Design review of the part shown in the three views and the two pictorial views. Dimensions are in mm from the part's minimum x, y and z. Round coordinates to 2 decimals unless told otherwise and drop trailing zeros. Loops run counter-clockwise (first coordinate to the right, second up) from the corner with the lowest first, then second, coordinate; pieces in that order, holes last.
1. Consider section B-B on x = 12.7. State the section outline as (y, z) points.
2. Clearance check with a flat-ended pin moving along its axis: pin 1 Ø4 at (x, y) = (63.5, 12.7) entering from -Z. State where the tip first meets the part, or that it passes through.
3. Consider section A-A on y = 38.1. State the section outline as (x, z) points.
4. To check wall thickness, follow line 1 along Y through (x, z) = (38.1, 2.5); line 2 along Y through (x, z) = (10, 0.75) (1 decimal); line 3 along X through (y, z) = (13.5, 1.75). State the ranges of each line that lie inside material, in increasing order.
5. Consider section D-D on z = 1. State how many separate pieces and enclosed holes the cut face has, then the cut area to 3 significant figures.
6. Consider section C-C on y = 63.5. State the section outline as (x, z) points.
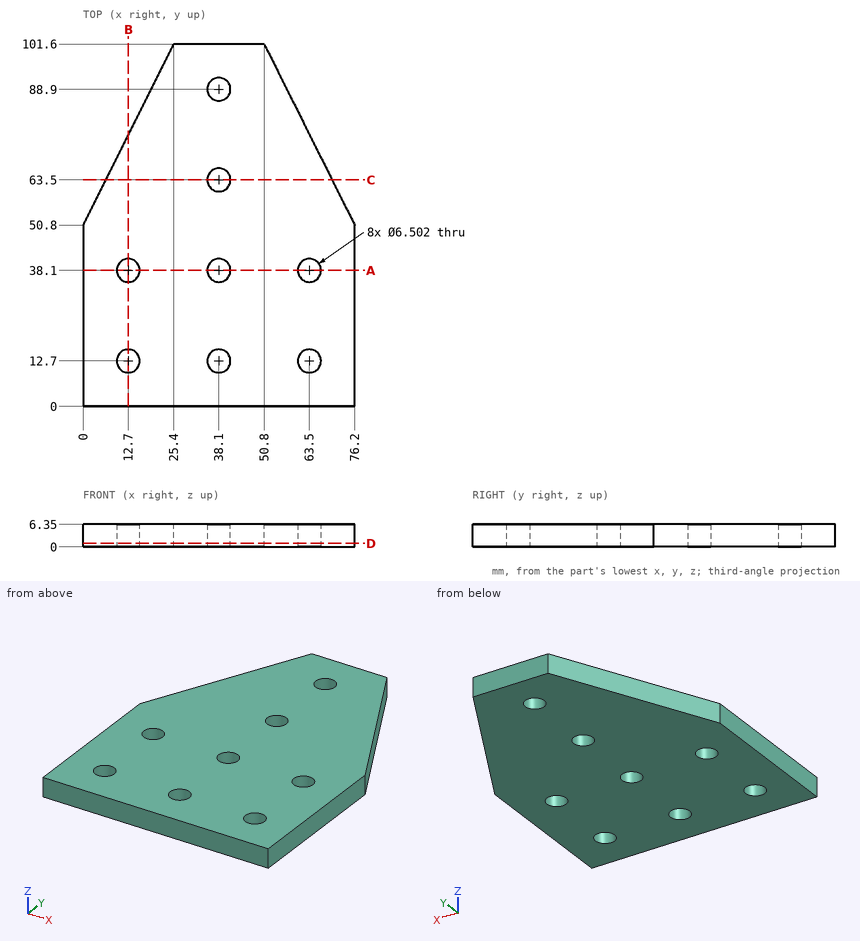
Resolved:
1. outline: (0, 0) - (9.45, 0) - (9.45, 6.35) - (0, 6.35) - close; (15.95, 0) - (34.85, 0) - (34.85, 6.35) - (15.95, 6.35) - close; (41.35, 0) - (76.2, 0) - (76.2, 6.35) - (41.35, 6.35) - close
2. pin 1: passes through
3. outline: (0, 0) - (9.45, 0) - (9.45, 6.35) - (0, 6.35) - close; (15.95, 0) - (34.85, 0) - (34.85, 6.35) - (15.95, 6.35) - close; (41.35, 0) - (60.25, 0) - (60.25, 6.35) - (41.35, 6.35) - close; (66.75, 0) - (76.2, 0) - (76.2, 6.35) - (66.75, 6.35) - close
4. line 1: y = 0 to 9.45, 15.95 to 34.85, 41.35 to 60.25, 66.75 to 85.65, 92.15 to 101.6
4. line 2: y = 0 to 10.9, 14.5 to 36.3, 39.9 to 70.8
4. line 3: x = 0 to 9.55, 15.85 to 34.95, 41.25 to 60.35, 66.65 to 76.2
5. separate pieces: 1
5. enclosed holes: 8
5. area: 6,190 mm2
6. outline: (6.35, 0) - (34.85, 0) - (34.85, 6.35) - (6.35, 6.35) - close; (41.35, 0) - (69.85, 0) - (69.85, 6.35) - (41.35, 6.35) - close
